Check sheet for the drawn part. Datum: minimum x, y, z corner. Units: mm. Coordinates: 2 decimals unless noted, no trailing zeros. Write each loop counter-clockwise with the first axis right and the second up, starting at its lowest first coordinate (ties: lowest second). Pieces come first, ordered by that corner, then holes. Notation, with made-up numbers: M -12,20.25 L 25,20.25 A9 ccw 25,33.25 Z; hole C 77.5,-35.5 d4. An arc over 180 degrees is marked long. Write item = value, one per line. Start each with the question number.
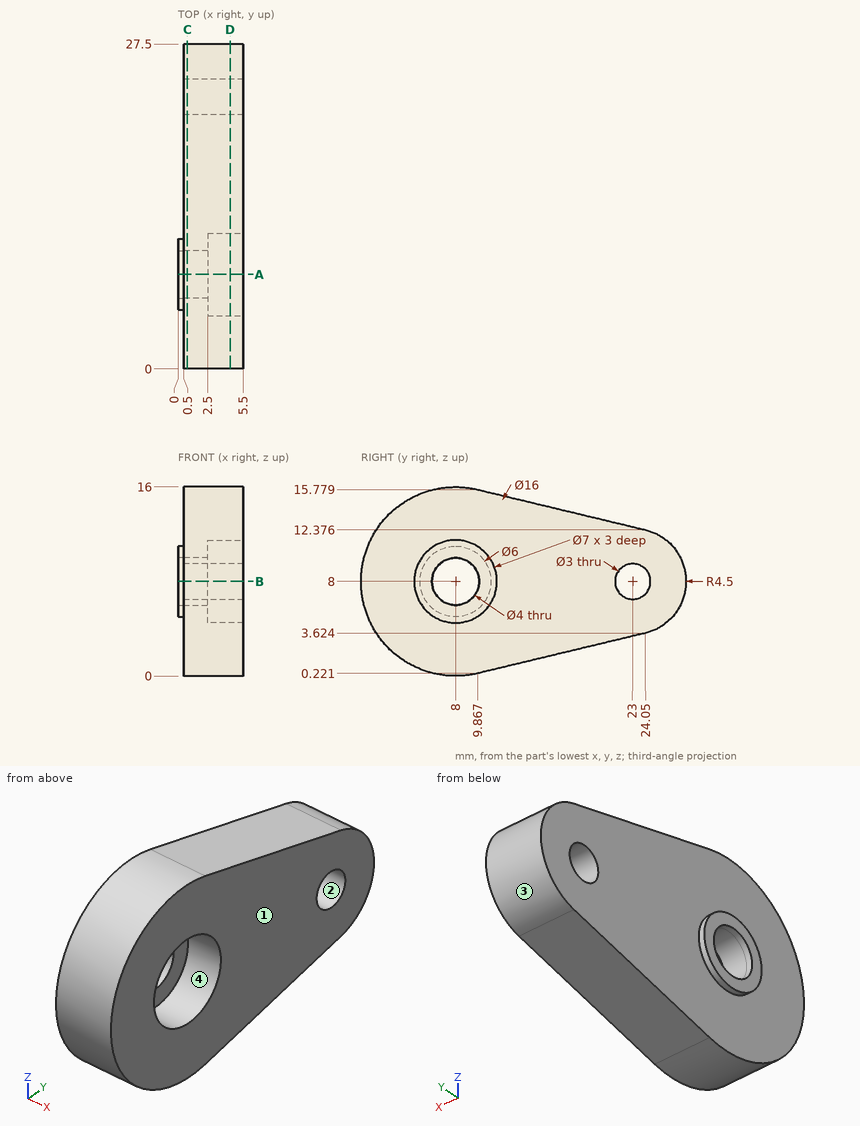
Q1. Gauge pin test, flat ends, axial feed: pin 1 (3 mm diameter, centred on x = 3.5, z = 12, fed in from +Y); pin 2 (6 mm diameter, centred on y = 17, z = 4.5, fed in from -X); pin 3 (5 mm diameter, centred on y = 10, z = 11, fed in from -X); pin 4 (4.5 mm diameter, centred on y = 8, z = 8, fed in from +X). Record the tip position at first contact, or that the pin passes through.
Q2. Cross-section at B-B on z = 8. Enter the section's corners in (x, y), and give its area (3 significant figures).
Q3. Cross-section at A-A on y = 8. Enter the section's corners in (x, z), and give its area (3 significant figures).
Q4. Cross-section at D-D on x = 4.4. Enter the section's corners in (y, z), and give its area (3 significant figures).
Q5. Draft check along Z on the marked faces 1, 2, 3 and 4. Enter one of: pulls with the +Z half, pulls with the -Z half, needs draft (parallel to the pull), parting line crosses it, or undercut.
Q6. Scan lines: L1, parallel to X at y = 13.5, z = 1.75; L2, parallel to Z at x = 1.45, y = 9.25; L3, parallel to Z at x = 1.35, y = 8.75 (1 decimal). Record each from-to range of solid material in increasing order.
Q7. Cross-section at C-C on x = 0.8. Enter the section's corners in (y, z).
Values found:
q1.pin_1 = 26.74
q1.pin_2 = 0.5
q1.pin_3 = 0
q1.pin_4 = 2.5
q2.outline = M 0,5 L 0.5,5 L 0.5,0 L 5.5,0 L 5.5,4.5 L 2.5,4.5 L 2.5,6 L 0,6 Z; M 0,10 L 2.5,10 L 2.5,11.5 L 5.5,11.5 L 5.5,21.5 L 0.5,21.5 L 0.5,11 L 0,11 Z; M 0.5,24.5 L 5.5,24.5 L 5.5,27.5 L 0.5,27.5 Z
q2.area = 94.5 mm²
q3.outline = M 0,5 L 0.5,5 L 0.5,0 L 5.5,0 L 5.5,4.5 L 2.5,4.5 L 2.5,6 L 0,6 Z; M 0,10 L 2.5,10 L 2.5,11.5 L 5.5,11.5 L 5.5,16 L 0.5,16 L 0.5,11 L 0,11 Z
q3.area = 52.0 mm²
q4.outline = M 9.87,0.22 L 24.05,3.62 A4.5 ccw 24.05,12.38 L 9.87,15.78 A8 ccw long Z; hole C 8,8 d7; hole C 23,8 d3
q4.area = 279 mm²
q5.face_1 = needs draft
q5.face_2 = undercut
q5.face_3 = parting line crosses it
q5.face_4 = undercut
q6.L1 = 0.5 to 5.5
q6.L2 = 0.1 to 6.44, 9.56 to 15.9
q6.L3 = 0 to 6.1, 9.9 to 16
q7.outline = M 9.87,0.22 L 24.05,3.62 A4.5 ccw 24.05,12.38 L 9.87,15.78 A8 ccw long Z; hole C 8,8 d4; hole C 23,8 d3
